CAD build for the part. Positions are in the model's coordinates, mm. Face numbers are marked on the shaded views. Give positions to 0.01 mm unless a question says otherwise; leave off trailing zeros. Order: outer loops, then holes, each group sorted by start corner. A loop starts at its lowest first (then second) coordinate and runs counter-clockwise, first axis right, second up.
Item 1: Band-saw the part on A-A on y = 25.4. Give the cut face in (x, z) (3 decimals), plus the area to 3 significant figures.
Item 2: Flat gauge pins, fed straight in: P1, Ø1, axis at x = 11, z = 2, coming from the +Y side; P2, Ø1.8, axis at y = 25.5, z = 3.5, coming from the -X side; P3, Ø1.8, axis at y = 32.5, z = 3, coming from the +X side (3 decimals); P4, Ø4, axis at x = 15, y = 24, coming from the +Z side. Where does each tip first touch, or does it go through?
Item 3: Wall check: L1, parallel to Z at x = 1.5, y = 34; L2, parallel to Z at x = -2.25, y = 18.5; L3, parallel to X at y = 19.5, z = 2.75 (3 decimals). Give the ranges that are in metal, low to high.
Item 4: Band-saw the part on C-C on z = 3.25. Give the cut face in (x, y) (3 decimals).
Item 5: Two-plate mould, pull along Z, no slides. Class the marked faces 1 and 2: released by +Z, released by -Z, zero draft, split by the parting line, or undercut.
Item 6: Band-saw the part on B-B on y = 9.5. Give the cut face in (x, z) (3 decimals), plus the area to 3 significant figures.
```python
from build123d import *

# Parameters (mm, degrees)
BOSS_EXTRUDE1_DEPTH = 50.8
CUT_EXTRUDE1_DEPTH  = 2.27


with BuildPart() as part:
    # Sketch2 → Boss-Extrude1 (new body)
    with BuildSketch(Plane(origin=(0, 0, 0), x_dir=(1, 0, 0), z_dir=(0, 1, 0))):
        with BuildLine():
            Line((-5.969, 0), (19.431, 0))
            ThreePointArc((19.431, 0), (19.700407684, -0.111592316), (19.812, -0.381))
            Line((19.812, -0.381), (19.812, -0.889))
            ThreePointArc((19.812, -0.889), (19.700407684, -1.158407684), (19.431, -1.27))
            Line((19.431, -1.27), (1.016, -1.27))
            ThreePointArc((1.016, -1.27), (0.746592316, -1.381592316), (0.635, -1.651))
            Line((0.635, -1.651), (0.635, -3.937))
            ThreePointArc((0.635, -3.937), (0.746592316, -4.206407684), (1.016, -4.318))
            Line((1.016, -4.318), (1.40496875, -4.318))
            ThreePointArc((1.40496875, -4.318), (1.539672592, -4.293392866), (1.656976563, -4.22275))
            ThreePointArc((1.656976563, -4.22275), (3.556, -5.08), (1.656976563, -5.93725))
            ThreePointArc((1.656976563, -5.93725), (1.539672592, -5.866607134), (1.40496875, -5.842))
            Line((1.40496875, -5.842), (-1.40496875, -5.842))
            ThreePointArc((-1.40496875, -5.842), (-1.539672592, -5.866607134), (-1.656976563, -5.93725))
            ThreePointArc((-1.656976563, -5.93725), (-3.556, -5.08), (-1.656976563, -4.22275))
            ThreePointArc((-1.656976563, -4.22275), (-1.539672592, -4.293392866), (-1.40496875, -4.318))
            Line((-1.40496875, -4.318), (-1.016, -4.318))
            ThreePointArc((-1.016, -4.318), (-0.746592316, -4.206407684), (-0.635, -3.937))
            Line((-0.635, -3.937), (-0.635, -1.651))
            ThreePointArc((-0.635, -1.651), (-0.746592316, -1.381592316), (-1.016, -1.27))
            Line((-1.016, -1.27), (-5.969, -1.27))
            ThreePointArc((-5.969, -1.27), (-6.238407684, -1.158407684), (-6.35, -0.889))
            Line((-6.35, -0.889), (-6.35, -0.381))
            ThreePointArc((-6.35, -0.381), (-6.238407684, -0.111592316), (-5.969, 0))
        make_face()
    extrude(amount=BOSS_EXTRUDE1_DEPTH)

    # Sketch3 → Cut-Extrude1 (cut, through all)
    with BuildSketch(Plane.XY.offset(1.27)):
        with BuildLine():
            Line((8.2931, 27.3812), (9.8806, 27.3812))
            Line((9.8806, 27.3812), (9.8806, 28.9814))
            ThreePointArc((9.8806, 28.9814), (11.8618, 30.9626), (13.843, 28.9814))
            Line((13.843, 28.9814), (13.843, 27.3812))
            Line((13.843, 27.3812), (15.4305, 27.3812))
            ThreePointArc((15.4305, 27.3812), (17.4117, 25.4), (15.4305, 23.4188))
            Line((15.4305, 23.4188), (8.2931, 23.4188))
            ThreePointArc((8.2931, 23.4188), (6.3119, 25.4), (8.2931, 27.3812))
        make_face()
    extrude(amount=-CUT_EXTRUDE1_DEPTH, mode=Mode.SUBTRACT)


solid = part.part
```
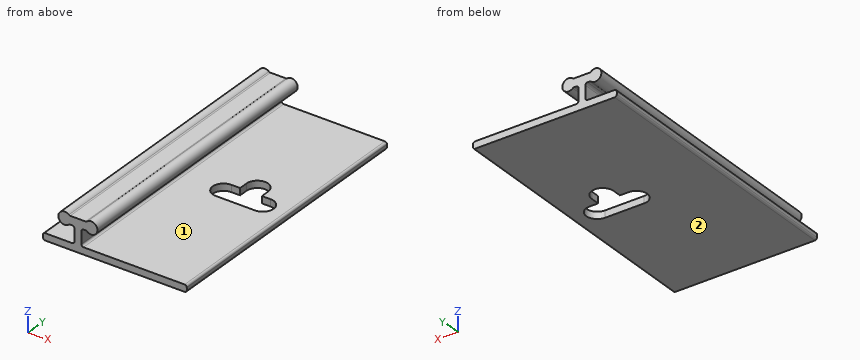
The answers:
1. outline: (-6.35, 0.381) arc R0.381 ccw to (-5.969, 0) - (6.312, 0) - (6.312, 1.27) - (1.016, 1.27) arc R0.381 cw to (0.635, 1.651) - (0.635, 3.937) arc R0.381 cw to (1.016, 4.318) - (1.405, 4.318) arc R0.381 cw to (1.657, 4.223) arc R1.143 ccw (long way) to (1.657, 5.937) arc R0.381 cw to (1.405, 5.842) - (-1.405, 5.842) arc R0.381 cw to (-1.657, 5.937) arc R1.143 ccw (long way) to (-1.657, 4.223) arc R0.381 cw to (-1.405, 4.318) - (-1.016, 4.318) arc R0.381 cw to (-0.635, 3.937) - (-0.635, 1.651) arc R0.381 cw to (-1.016, 1.27) - (-5.969, 1.27) arc R0.381 ccw to (-6.35, 0.889) - close; (17.412, 0) - (19.431, 0) arc R0.381 ccw to (19.812, 0.381) - (19.812, 0.889) arc R0.381 ccw to (19.431, 1.27) - (17.412, 1.27) - close
1. area: 35.4 mm2
2. P1: passes through
2. P2: stops at x = -3.33
2. P3: stops at x = 0.635
2. P4: stops at z = 1.27
3. L1: z = 0 to 1.27, 4.31 to 5.85
3. L2: z = 0 to 1.27, 3.95 to 6.21
3. L3: x = -0.635 to 0.635
4. outline: (-0.635, 0) - (0.635, 0) - (0.635, 50.8) - (-0.635, 50.8) - close
5. face 1: undercut
5. face 2: released by -Z
6. outline: (-6.35, 0.381) arc R0.381 ccw to (-5.969, 0) - (19.431, 0) arc R0.381 ccw to (19.812, 0.381) - (19.812, 0.889) arc R0.381 ccw to (19.431, 1.27) - (1.016, 1.27) arc R0.381 cw to (0.635, 1.651) - (0.635, 3.937) arc R0.381 cw to (1.016, 4.318) - (1.405, 4.318) arc R0.381 cw to (1.657, 4.223) arc R1.143 ccw (long way) to (1.657, 5.937) arc R0.381 cw to (1.405, 5.842) - (-1.405, 5.842) arc R0.381 cw to (-1.657, 5.937) arc R1.143 ccw (long way) to (-1.657, 4.223) arc R0.381 cw to (-1.405, 4.318) - (-1.016, 4.318) arc R0.381 cw to (-0.635, 3.937) - (-0.635, 1.651) arc R0.381 cw to (-1.016, 1.27) - (-5.969, 1.27) arc R0.381 ccw to (-6.35, 0.889) - close
6. area: 49.5 mm2
